from build123d import *

# Parameters (mm, degrees)
SKETCH009_R   = 2.5
PAD009_DEPTH  = 4.2
SKETCH010_R   = 2.5
SKETCH010_R_2 = 3.15
PAD010_DEPTH  = 4
SKETCH011_R   = 4.6
HOLE_DEPTH    = 2
HOLE_TIPS_R   = 4.6


with BuildPart() as part:
    # Sketch009 → Pad009 (new body)
    with BuildSketch(Plane.XY):
        with BuildLine():
            Line((-9, 30), (-9, -30))
            ThreePointArc((-9, -30), (-8.12132, -32.12132), (-6, -33))
            Line((-6, -33), (6, -33))
            ThreePointArc((6, -33), (8.12132, -32.12132), (9, -30))
            Line((9, -30), (9, 30))
            ThreePointArc((9, 30), (8.12132, 32.12132), (6, 33))
            Line((6, 33), (-6, 33))
            ThreePointArc((-6, 33), (-8.12132, 32.12132), (-9, 30))
        make_face()
        with Locations((0, 27.5)):
            Circle(SKETCH009_R, mode=Mode.SUBTRACT)
        with Locations((0, -27.5)):
            Circle(SKETCH009_R, mode=Mode.SUBTRACT)
        Circle(SKETCH009_R, mode=Mode.SUBTRACT)
        Polygon((3.002221, 11.3), (6.004443, 16.5), (3.002221, 21.7), (-3.002221, 21.7), (-6.004443, 16.5), (-3.002221, 11.3), align=None, mode=Mode.SUBTRACT)
        Polygon((-3.002221, -21.7), (3.002221, -21.7), (6.004443, -16.5), (3.002221, -11.3), (-3.002221, -11.3), (-6.004443, -16.5), align=None, mode=Mode.SUBTRACT)
    extrude(amount=PAD009_DEPTH)

    # Sketch010 (on Face25 of Pad009) → Pad010 (join)
    with BuildSketch(Plane.XY.offset(4.2)):
        with BuildLine():
            Line((-9, 30), (-9, -30))
            ThreePointArc((-9, -30), (-8.12132, -32.12132), (-6, -33))
            Line((-6, -33), (6, -33))
            ThreePointArc((6, -33), (8.12132, -32.12132), (9, -30))
            Line((9, -30), (9, 30))
            ThreePointArc((9, 30), (8.12132, 32.12132), (6, 33))
            Line((6, 33), (-6, 33))
            ThreePointArc((-6, 33), (-8.12132, 32.12132), (-9, 30))
        make_face()
        with Locations((0, 27.5)):
            Circle(SKETCH010_R, mode=Mode.SUBTRACT)
        Circle(SKETCH010_R, mode=Mode.SUBTRACT)
        with Locations((0, -27.5)):
            Circle(SKETCH010_R, mode=Mode.SUBTRACT)
        with Locations((0, 16.5)):
            Circle(SKETCH010_R_2, mode=Mode.SUBTRACT)
        with Locations((0, -16.5)):
            Circle(SKETCH010_R_2, mode=Mode.SUBTRACT)
    extrude(amount=PAD010_DEPTH)

    # Sketch011 (on Face17 of Pad010) → Hole (cut)
    with BuildSketch(Plane.XY.offset(8.2)):
        Circle(SKETCH011_R)
        with Locations((0, -27.5)):
            Circle(SKETCH011_R)
        with Locations((0, 27.5)):
            Circle(SKETCH011_R)
    extrude(amount=-HOLE_DEPTH, mode=Mode.SUBTRACT)

    # Hole tips → Hole tip 1 section 0
    with BuildSketch(Plane.XY.offset(6.2), mode=Mode.PRIVATE) as hole_tip_1_s0:
        Circle(HOLE_TIPS_R)
    loft([hole_tip_1_s0.sketch, Vertex(0, 0, 1.6)], mode=Mode.SUBTRACT)

    # Hole tips → Hole tip 2 section 0
    with BuildSketch(Plane.XY.offset(6.2), mode=Mode.PRIVATE) as hole_tip_2_s0:
        with Locations((0, -27.5)):
            Circle(HOLE_TIPS_R)
    loft([hole_tip_2_s0.sketch, Vertex(0, -27.5, 1.6)], mode=Mode.SUBTRACT)

    # Hole tips → Hole tip 3 section 0
    with BuildSketch(Plane.XY.offset(6.2), mode=Mode.PRIVATE) as hole_tip_3_s0:
        with Locations((0, 27.5)):
            Circle(HOLE_TIPS_R)
    loft([hole_tip_3_s0.sketch, Vertex(0, 27.5, 1.6)], mode=Mode.SUBTRACT)


solid = part.part
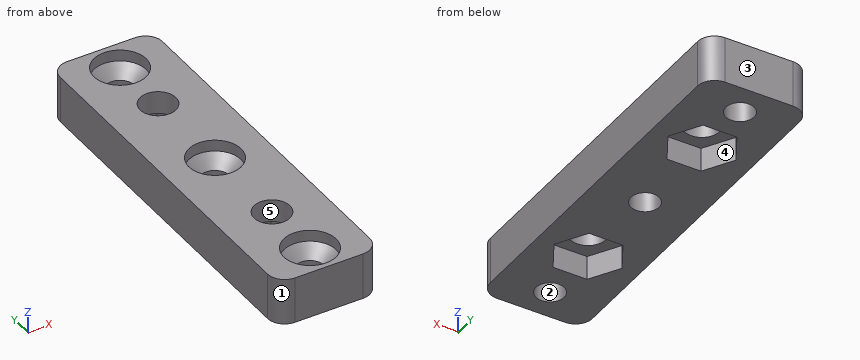
Build history of the part. All positions in model axes, mm. Face numbers are marked on the shaded views. A direction names the side the tool comes from. Round coordinates to 2 decimals unless told otherwise and drop trailing zeros. Write each loop counter-clockwise with the first axis right and the second up, starting at its lowest first coordinate (ties: lowest second). Pieces come first, ordered by that corner, then holes. Notation, with made-up numbers: (-0.5, -31) - (56.5, -31) arc R9 cw to (56.5, -25) - close; hole circle Ø7 at (80, 72.5). An arc over 180 degrees is marked (long way). One line per question, with ' | ' between items.
1. Drill centre lines: line 1 along Y through (x, z) = (0, 2.15); line 2 along Y through (x, z) = (0, 6.65); line 3 along Y through (x, z) = (-3.75, 1). Where is each one in solid material? Low to high. Write a range as from..to.
Results are:
line 1: -33..-30, -25..-21.7, -11.3..-2.5, 2.5..11.3, 21.7..25, 30..33 | line 2: -33..-32.1, -22.9..-19.65, -13.35..-4.6, 4.6..13.35, 19.65..22.9, 32.1..33 | line 3: -33..-20.4, -12.6..12.6, 20.4..33
2. Band-saw the part on C-C, the plane y = -20.5. Write the cut outline in (x, z).
Results are:
outline: (-9, 0) - (-3.7, 0) - (-3.7, 4.2) - (3.7, 4.2) - (3.7, 0) - (9, 0) - (9, 8.2) - (-9, 8.2) - close
3. Tool access for the marked faces 4 and 5: list every direction of +Z, -Z, +X, -X, +Y, -Y with a clear straight run to the whole face (end or side of a thin tool).
Results are:
face 4: -Z | face 5: +Z, -Z
4. Drop a flat-ended pin along its axis: pin 1 Ø7 at (x, y) = (0, 16.5) entering from -Z. Give the stop position or say it passes through.
Results are:
pin 1: z = 4.2
5. Mould opens along Y. For the marked faces 1, 2 and 3 say: released by +Y, released by -Y, zero draft, split by the parting line, or undercut.
Results are:
face 1: released by -Y | face 2: undercut | face 3: released by +Y
6. Band-saw the part on B-B, the plane z = 2. Write the cut outline in (x, y), and give its area (3 significant figures).
Results are:
outline: (-9, -30) arc R3 ccw to (-6, -33) - (6, -33) arc R3 ccw to (9, -30) - (9, 30) arc R3 ccw to (6, 33) - (-6, 33) arc R3 ccw to (-9, 30) - close; hole (-6, -16.5) - (-3, -21.7) - (3, -21.7) - (6, -16.5) - (3, -11.3) - (-3, -11.3) - close; hole (-6, 16.5) - (-3, 11.3) - (3, 11.3) - (6, 16.5) - (3, 21.7) - (-3, 21.7) - close; hole circle Ø5 at (0, -27.5); hole circle Ø5 at (0, 0); hole circle Ø5 at (0, 27.5) | area: 934 mm^2
7. Band-saw the part on A-A, the plane z = 5. Write the cut outline in (x, y).
Results are:
outline: (-9, -30) arc R3 ccw to (-6, -33) - (6, -33) arc R3 ccw to (9, -30) - (9, 30) arc R3 ccw to (6, 33) - (-6, 33) arc R3 ccw to (-9, 30) - close; hole circle Ø6.8 at (0, -27.5); hole circle Ø6.8 at (0, 0); hole circle Ø6.8 at (0, 27.5); hole circle Ø6.3 at (0, -16.5); hole circle Ø6.3 at (0, 16.5)
